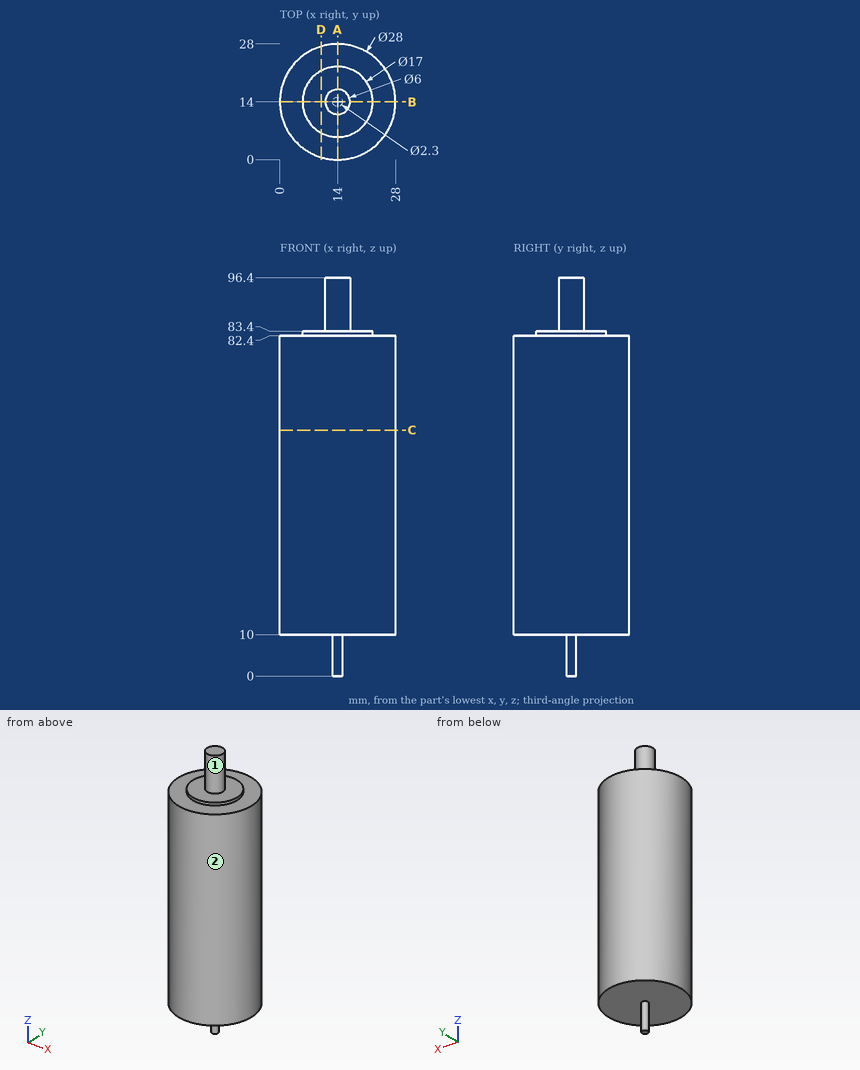
Verification items for this drawing (mm, ordinates from the low corner). A direction names the side the tool comes from. Coordinates: 2 decimals unless noted, no trailing zeros. Order: outer loops, then holes, each group sorted by start corner. A loop starts at its lowest first (then second) coordinate and runs counter-clockwise, first axis right, second up.
Q1. Depth check by flat-ended pin: pin 1 Ø1 at (x, z) = (8.5, 67.5) entering from +Y; pin 2 Ø6 at (y, z) = (4, 15) entering from -X; pin 3 Ø10 at (y, z) = (24.5, 50.5) entering from -X. Enter the tip coordinate at first touch or a pass-through.
Reply:
pin 1: stops at y = 27.08
pin 2: stops at x = 1.88
pin 3: stops at x = 1.13
Q2. Sectioned sample at C-C on z = 59.5. Record the cut outline in (x, y).
Reply:
outline: circle Ø28 at (14, 14)
Q3. Tool access check on the marked faces 1 and 2. Record the directions out of +Z, -Z, +X, -X, +Y, -Y that give a thin tool (end or side, any length) a straight path to the whole face; none if there is none.
Reply:
face 1: +Z
face 2: +Z, -Z
Q4. Sectioned sample at A-A on x = 14. Record the cut outline in (y, z).
Reply:
outline: (0, 10) - (12.85, 10) - (12.85, 0) - (15.15, 0) - (15.15, 10) - (28, 10) - (28, 82.4) - (22.5, 82.4) - (22.5, 83.4) - (17, 83.4) - (17, 96.4) - (11, 96.4) - (11, 83.4) - (5.5, 83.4) - (5.5, 82.4) - (0, 82.4) - close
Q5. Sectioned sample at D-D on x = 10. Record the cut outline in (y, z), and give its area (3 significant figures).
Reply:
outline: (0.58, 10) - (27.42, 10) - (27.42, 82.4) - (21.5, 82.4) - (21.5, 83.4) - (6.5, 83.4) - (6.5, 82.4) - (0.58, 82.4) - close
area: 1,960 mm2
Q6. Thickness scan on probe 1 along Z at (x, y) = (1, 15); probe 2 along Z at (x, y) = (11.75, 7.75); probe 3 along X at (y, z) = (14.5, 38.5). Record the ranges inside material, lowest first.
Reply:
probe 1: z = 10 to 82.4
probe 2: z = 10 to 83.4
probe 3: x = 0.01 to 27.99
